Part model, mm, in its own coordinate system. Round coordinates to 2 decimals unless told otherwise and drop trailing zeros. Order: outer loops, then holes, each group sorted by start corner. A loop starts at its lowest first (then second) coordinate and runs counter-clockwise, first axis right, second up. Notation, with made-up numbers: (8.25, -2.75) - (41.25, -2.75) arc R30 cw to (41.25, 35.25) - close; hole circle Ø1 at (-18.75, -19.5). An arc over 180 degrees is marked (long way). Return JSON: item names as keys, results as strings. Group by question number.
Item 1: Probe probe 1 along Z at (x, y) = (8.5, -21); probe 2 along Y at (x, z) = (11, 114); probe 3 along Y at (x, z) = (14.75, 34). List the from-to ranges inside material, lowest first.
Item 2: Drop a flat-ended pin along its axis: pin 1 (6 mm diameter, centred on x = 5, y = -68, fed in from -Z). Give the stop position or say it passes through.
Item 3: Saw through at A-A on x = 11.5. List the corners of the cut face in (y, z).
Item 4: Saw through at B-B on z = 117.5. List the corners of the cut face in (x, y).
Item 5: Saw through at C-C on y = -153. List the corners of the cut face in (x, z).
```python
from build123d import *

# Parameters (mm, degrees)
PAD_DEPTH = 18


with BuildPart() as part:
    # Sketch → Pad (new body)
    with BuildSketch(Plane.YZ):
        Polygon((0, 170), (-170, 170), (-170, 150), (-20, 0), (0, 0), align=None)
    extrude(amount=PAD_DEPTH)


solid = part.part
```
Filled in:
{
 "1": {"probe 1": "z = 1 to 170", "probe 2": "y = -134 to 0", "probe 3": "y = -54 to 0"},
 "2": {"pin 1": "stops at z = 45"},
 "3": {"outline": "(-170, 150) - (-20, 0) - (0, 0) - (0, 170) - (-170, 170) - close"},
 "4": {"outline": "(0, -137.5) - (18, -137.5) - (18, 0) - (0, 0) - close"},
 "5": {"outline": "(0, 133) - (18, 133) - (18, 170) - (0, 170) - close"}
}
